Autodesk Fusion 360 part; units mm, degrees
sketch "Sketch1" plane through (0, 0, 0) normal (0, 0, 1) x (1, 0, 0)
  line L0 (-40, -50) -> (589, -50)
  line L1 (589, -50) -> (589, 274)
  line L2 (589, 274) -> (-40, 274)
  line L3 (-40, 274) -> (-40, -50)
  circle A0 centre (583.5, -44.5) radius 5
  circle A1 centre (583.5, 268.5) radius 5
  circle A2 centre (-34.5, 268.5) radius 5
  circle A3 centre (-34.5, -44.5) radius 5
  line L4 (-30, 250) -> (-5, 250)
  line L5 (-5, 250) -> (-5, -25)
  line L6 (-5, -25) -> (-30, -25)
  line L7 (-30, -25) -> (-30, 250)
  line L8 (579, 250) -> (554, 250)
  line L9 (554, 250) -> (554, -25)
  line L10 (554, -25) -> (579, -25)
  line L11 (579, -25) -> (579, 250)
  dimension "d1" = 629
  dimension "d2" = 324
  dimension "d3" = 10
  dimension "d4" = 5.5
  dimension "d5" = 5.5
  dimension "d6" = 10
  dimension "d7" = 5.5
  dimension "d8" = 5.5
  dimension "d9" = 10
  dimension "d10" = 5.5
  dimension "d11" = 5.5
  dimension "d12" = 10
  dimension "d13" = 5.5
  dimension "d14" = 5.5
  dimension "d15" = 10
  dimension "d16" = 559
extrude "Extrude1" add sketch "Sketch1" along normal blind 5
extrude "Extrude2" add sketch "Sketch1" along normal blind 48 contours L4 L5 L6 L7 | L8 L9 L10 L11
extrude "Extrude3" add sketch "Sketch1" along normal blind 55 contours A3
extrude "Extrude4" add sketch "Sketch1" along normal blind 55 contours A2
extrude "Extrude5" add sketch "Sketch1" along normal blind 55 contours A1
extrude "Extrude6" add sketch "Sketch1" along normal blind 55 contours A0
Source: CAD feature listing. Evaluate the final solid. Frame: model axes, mm. Coordinates: 2 decimals unless noted, no trailing zeros. Write each loop counter-clockwise with the first axis right and the second up, starting at its lowest first coordinate (ties: lowest second). Pieces come first, ordered by that corner, then holes. Notation, with made-up numbers: (-38.5, 7) -> (1.5, 7) arc R6 cw to (1.5, 16) -> close; hole circle Ø10 at (15, -6). An arc over 180 degrees is marked (long way). Return JSON: item names as keys, results as strings. Group by question number.
1) Mould query, pull axis X, two halves, no side actions, for faces 1 (the face through (-30, 111, 26)), 2 (the face through (554, 114, 26)), 3 (the face through (270, 114, 0)), 4 (the face through (579, 111, 26)). Classes: +X half, -X half, draft (parallel to the pull), parting line (faces both ways), or undercut.
2) Section query B-B, the plane y = 172. Return loops of the section in (x, z).
3) Section query A-A, the plane z = 32.5. Return loops of the section in (x, y), plus the area to 3 significant figures.
4) Contact query for flat-ended pins moving along their axis: P1, Ø21.5, axis at y = 45.5, z = 34.5, coming from the -X side; P2, Ø12.5, axis at x = -20.5, z = 35, coming from the -Y side; P3, Ø8, axis at y = 163.5, z = 16, coming from the +X side. Output: stop coordinate, or through.
5) Section query C-C, the plane x = 259.5. Return loops of the section in (y, z).
6) Ray query, line 1 along X through (y, z) = (10, 13.5); line 2 along Y through (x, z) = (-13.5, 11.5); line 3 along Z through (x, y) = (236.5, 55.5). Return the intervals inside material, ascending.
From the geometry:
{
 "1": {"face 1": "-X half", "face 2": "undercut", "face 3": "draft", "face 4": "+X half"},
 "2": {"outline": "(-40, 0) -> (589, 0) -> (589, 5) -> (579, 5) -> (579, 48) -> (554, 48) -> (554, 5) -> (-5, 5) -> (-5, 48) -> (-30, 48) -> (-30, 5) -> (-40, 5) -> close"},
 "3": {"outline": "circle Ø10 at (-34.5, -44.5); circle Ø10 at (-34.5, 268.5); (-30, -25) -> (-5, -25) -> (-5, 250) -> (-30, 250) -> close; (554, -25) -> (579, -25) -> (579, 250) -> (554, 250) -> close; circle Ø10 at (583.5, -44.5); circle Ø10 at (583.5, 268.5)", "area": "14,100 mm²"},
 "4": {"P1": "x = -30", "P2": "y = -25", "P3": "x = 579"},
 "5": {"outline": "(-50, 0) -> (274, 0) -> (274, 5) -> (-50, 5) -> close"},
 "6": {"line 1": "-30 to -5, 554 to 579", "line 2": "-25 to 250", "line 3": "0 to 5"}
}
